```python
from build123d import *

# Parameters (mm, degrees)
PAD_DEPTH            = 10
SKETCH005_R          = 1.6
POCKET001_DEPTH      = 6.001
POCKET001_DEPTH_BACK = -6.001
SKETCH_W             = 3
SKETCH_H             = 15
PAD001_DEPTH         = 10
SKETCH006_R          = 1.6
POCKET_DEPTH         = 8.001
POCKET_DEPTH_BACK    = 11.747425


with BuildPart() as part:
    # Sketch003 → Pad (new body)
    with BuildSketch(Plane.XZ):
        with BuildLine():
            Line((8, -6), (-11.746425, -6))
            Line((-11.746425, -2.8), (-11.746425, -6))
            Line((-1.746425, -2.8), (-11.746425, -2.8))
            ThreePointArc((-1.746425, -2.8), (3.3, 0), (-1.746425, 2.8))
            Line((-1.746425, 2.8), (-11.746425, 2.8))
            Line((-11.746425, 2.8), (-11.746425, 6))
            Line((2, 6), (-11.746425, 6))
            ThreePointArc((8, 0), (6.242641, 4.242641), (2, 6))
            Line((8, 0), (8, -6))
        make_face()
    extrude(amount=PAD_DEPTH)

    # Sketch005 → Pocket001 (cut, two sides)
    with BuildSketch(Plane.XY) as pocket001_sk:
        with Locations((-7.5, -5)):
            Circle(SKETCH005_R)
    extrude(amount=-POCKET001_DEPTH, mode=Mode.SUBTRACT)
    extrude(pocket001_sk.sketch, amount=-POCKET001_DEPTH_BACK, mode=Mode.SUBTRACT)

    # Sketch → Pad001 (join)
    with BuildSketch(Plane.XZ):
        with Locations((6.5, -13.5)):
            Rectangle(SKETCH_W, SKETCH_H)
        with Locations((-1.5, -13.5)):
            Rectangle(SKETCH_W, SKETCH_H)
    extrude(amount=PAD001_DEPTH)

    # Sketch006 → Pocket (cut, two sides)
    with BuildSketch(Plane.YZ) as pocket_sk:
        with Locations((-5, -16)):
            Circle(SKETCH006_R)
    extrude(amount=POCKET_DEPTH, mode=Mode.SUBTRACT)
    extrude(pocket_sk.sketch, amount=-POCKET_DEPTH_BACK, mode=Mode.SUBTRACT)


solid = part.part
```
Can you work these out from the model? Positions are in its coordinate system, mm. A direction names the side the tool comes from. Give positions to 0.01 mm unless a question says otherwise; leave off trailing zeros. Write each loop counter-clockwise with the first axis right and the second up, starting at its lowest first coordinate (ties: lowest second). Pieces come first, ordered by that corner, then holes. Notation, with made-up numbers: (57, 69) -> (113, 69) arc R21 ccw to (113, 96) -> close; hole circle Ø5 at (62, 29.25). An arc over 180 degrees is marked (long way). One line per item, written item: value.
Q1. For P1, Ø3, axis at x = -7, y = -6.5, coming from the -Z side; P2, Ø5.5, axis at x = 0, z = 0, coming from the +Y side, each with a flat end and sliding along its axis, tell me the tip position at first contact or that it passes through.
Results found:
P1: stops at z = -6
P2: passes through
Q2. We'd pull the mould along Z, two halves only. Please class faces 5 (the face through (-9.1, -4.93, -4.38)), 6 (the face through (-2, -5, -21)), 7 (the face through (3.3, -4.9, -0.1)): +Z half, -Z half, draft (parallel to the pull), parting line (faces both ways), or undercut.
Results found:
face 5: draft
face 6: -Z half
face 7: undercut
Q3. Imagine slicing it at A-A on x = -2.25. Please give me the cut outline in (y, z).
Results found:
outline: (-10, -21) -> (0, -21) -> (0, -2.8) -> (-10, -2.8) -> close; (-10, 2.8) -> (0, 2.8) -> (0, 6) -> (-10, 6) -> close; hole circle Ø3.2 at (-5, -16)
Q4. Imagine slicing it at D-D on x = -4.5. Please give me the cut outline in (y, z).
Results found:
outline: (-10, -6) -> (0, -6) -> (0, -2.8) -> (-10, -2.8) -> close; (-10, 2.8) -> (0, 2.8) -> (0, 6) -> (-10, 6) -> close
Q5. Which directions (+Z, -Z, +X, -X, +Y, -Y) give clear straight access to the entire face, cutting with the end or side of a thin tool? Please do faces 1 (the face through (-3, -5, -14)), 2 (the face through (-11.746, -5, -4)), 3 (the face through (0, -5, -14)), 4 (the face through (-5.6, -4.9, 2.8)).
Results found:
face 1: -Z, -X, +Y, -Y
face 2: +Z, -Z, -X, +Y, -Y
face 3: -Z, +Y, -Y
face 4: -X, +Y, -Y
Q6. Please list where these lines run through material, in increasing order: line 1 (X direction, y = -9.5, z = -9.5); line 2 (Z direction, x = -6.5, y = -3.25); line 3 (Y direction, x = -7.5, z = -5.3). Write a range as [from, to].
Results found:
line 1: x = [-3, 0], [5, 8]
line 2: z = [-6, -2.8], [2.8, 6]
line 3: y = [-10, -6.6], [-3.4, 0]
Q7. Imagine slicing it at C-C on z = -9.5. Please give me the cut outline in (x, y).
Results found:
outline: (-3, -10) -> (0, -10) -> (0, 0) -> (-3, 0) -> close; (5, -10) -> (8, -10) -> (8, 0) -> (5, 0) -> close
Q8. Imagine slicing it at B-B on y = -5. Give the number of separate pieces and of enclosed holes in the cut face, and give its area (3 significant figures).
Results found:
separate pieces: 5
enclosed holes: 0
area: 195 mm^2
